Geometry check sheet. Reference: the model listing, model coordinates, mm. Face numbers are marked on the shaded views. A direction names the side the tool comes from. Round coordinates to 2 decimals unless told otherwise and drop trailing zeros. Write each loop counter-clockwise with the first axis right and the second up, starting at its lowest first coordinate (ties: lowest second). Pieces come first, ordered by that corner, then holes. Notation, with made-up numbers: M 83,60.25 L 90,60.25 A13 ccw 90,71.25 Z; hole C 59.25,18.5 d7. An arc over 180 degrees is marked long. Put each result on its own line as item: value. Start each with the question number.
(1) Gauge pin test, flat ends, axial feed: pin 1 (1.1 mm diameter, centred on x = 28.5, z = -20, fed in from +Y); pin 2 (3 mm diameter, centred on x = -14, z = 20, fed in from -Y); pin 3 (0.9 mm diameter, centred on y = 11.5, z = 28, fed in from -X); pin 4 (2 mm diameter, centred on x = 14, z = 23.5, fed in from +Y). Record the tip position at first contact, or that the pin passes through.
(2) Material ranges on probe 1 along X at (y, z) = (7.5, 3); probe 2 along Z at (x, y) = (-43.5, 9.75); probe 3 along Z at (x, y) = (43.5, 16), recorded low to high.
(3) Tool access check on the marked faces 5 and 6. Record the directions out of +Z, -Z, +X, -X, +Y, -Y that give a thin tool (end or side, any length) a straight path to the whole face; none if there is none.
(4) Section check C-C on x = 48.5. Record the cut outline in (y, z), then the cut area to 3 significant figures.
(5) Section check B-B on x = -11.1. Record the cut outline in (y, z), then the cut area to 3 significant figures.
(6) Section check A-A on x = 14. Record the cut outline in (y, z).
(7) Mould release check, pull along Z, two halves, no side actions. Record for the marked faces 1, 2, 3 and 4: pulls with the +Z half, pulls with the -Z half, needs draft (parallel to the pull), parting line crosses it, or undercut.
from build123d import *

# Parameters (mm, degrees)
BOSS_EXTRUDE1_DEPTH = 2
BOSS_EXTRUDE2_DEPTH = 16
SKETCH12_W          = 7
SKETCH12_H          = 7
BOSS_EXTRUDE5_DEPTH = 16
FILLET1_R           = 3
SKETCH13_R          = 1.3
CUT_EXTRUDE7_DEPTH  = 19
SKETCH14_R          = 2.5
SKETCH14_R_2        = 1.15
BOSS_EXTRUDE6_DEPTH = 14
SKETCH15_R          = 2.5
SKETCH15_R_2        = 1.3
BOSS_EXTRUDE7_DEPTH = 3
SKETCH16_W          = 9
SKETCH16_H          = 4.5
CUT_EXTRUDE8_DEPTH  = 4
SKETCH17_R          = 3.25
CUT_EXTRUDE9_DEPTH  = 13
SKETCH19_R          = 2.5
SKETCH19_R_2        = 1.15
BOSS_EXTRUDE8_DEPTH = 2.5
SKETCH20_R          = 3.1
SKETCH20_R_2        = 3
SKETCH20_W          = 4
SKETCH20_H          = 11
CUT_EXTRUDE10_DEPTH = 5
SKETCH21_R          = 1.15
CUT_EXTRUDE11_DEPTH = 3.5
SKETCH22_R          = 1.15
CUT_EXTRUDE12_DEPTH = 3.5


with BuildPart() as part:
    # Sketch1 → Boss-Extrude1 (new body)
    with BuildSketch(Plane(origin=(0, 0, 0), x_dir=(1, 0, 0), z_dir=(0, 1, 0))):
        with BuildLine():
            Line((70, 10), (70, -10))
            ThreePointArc((70, -10), (64.142135624, -24.142135624), (50, -30))
            Line((50, -30), (-50, -30))
            ThreePointArc((-50, -30), (-64.142135624, -24.142135624), (-70, -10))
            Line((-70, -10), (-70, 10))
            ThreePointArc((-70, 10), (-64.142135624, 24.142135624), (-50, 30))
            Line((-50, 30), (50, 30))
            ThreePointArc((50, 30), (64.142135624, 24.142135624), (70, 10))
        make_face()
    extrude(amount=BOSS_EXTRUDE1_DEPTH)

    # Sketch2 → Boss-Extrude2 (add)
    with BuildSketch(Plane(origin=(0, 2, 0), x_dir=(1, 0, 0), z_dir=(0, 1, 0))):
        with BuildLine():
            Line((-50, 30), (50, 30))
            ThreePointArc((50, 30), (64.142135624, 24.142135624), (70, 10))
            Line((70, 10), (70, -10))
            ThreePointArc((70, -10), (64.142135624, -24.142135624), (50, -30))
            Line((50, -30), (-50, -30))
            ThreePointArc((-50, -30), (-64.142135624, -24.142135624), (-70, -10))
            Line((-70, -10), (-70, 10))
            ThreePointArc((-70, 10), (-64.142135624, 24.142135624), (-50, 30))
        make_face()
        with BuildLine():
            Line((-47, 27), (47, 27))
            ThreePointArc((47, 27), (60.435028843, 21.435028843), (66, 8))
            Line((66, 8), (66, -12))
            ThreePointArc((66, -12), (59.103718437, -22.798043353), (47, -27))
            Line((47, -27), (-47, -27))
            ThreePointArc((-47, -27), (-59.103718437, -22.798043353), (-66, -12))
            Line((-66, -12), (-66, 8))
            ThreePointArc((-66, 8), (-60.435028843, 21.435028843), (-47, 27))
        make_face(mode=Mode.SUBTRACT)
    extrude(amount=BOSS_EXTRUDE2_DEPTH)

    # Sketch12 → Boss-Extrude5 (add)
    with BuildSketch(Plane(origin=(0, 2, 0), x_dir=(1, 0, 0), z_dir=(0, 1, 0))):
        with Locations((-43.5, 23.5)):
            Rectangle(SKETCH12_W, SKETCH12_H)
        with Locations((-43.5, -23.5)):
            Rectangle(SKETCH12_W, SKETCH12_H)
        with Locations((43.5, -23.5)):
            Rectangle(SKETCH12_W, SKETCH12_H)
        with Locations((43.5, 23.5)):
            Rectangle(SKETCH12_W, SKETCH12_H)
    extrude(amount=BOSS_EXTRUDE5_DEPTH)

    # Fillet1
    fillet1_edges = [part.edges().sort_by_distance(p)[0] for p in [
        (70, 0, 0),
        (64.142135624, 0, 24.142135624),
        (0, 0, 30),
        (-64.142135624, 0, 24.142135624),
        (-70, 0, 0),
        (-64.142135624, 0, -24.142135624),
        (0, 0, -30),
        (64.142135624, 0, -24.142135624),
    ]]
    fillet(fillet1_edges, radius=FILLET1_R)

    # Sketch13 → Cut-Extrude7 (cut, through all)
    with BuildSketch(Plane(origin=(0, 18, 0), x_dir=(1, 0, 0), z_dir=(0, 1, 0))):
        with Locations((-43.5, 23.5)):
            Circle(SKETCH13_R)
        with Locations((-43.5, -23.5)):
            Circle(SKETCH13_R)
        with Locations((43.5, -23.5)):
            Circle(SKETCH13_R)
        with Locations((43.5, 23.5)):
            Circle(SKETCH13_R)
    extrude(amount=-CUT_EXTRUDE7_DEPTH, mode=Mode.SUBTRACT)

    # Sketch14 → Boss-Extrude6 (add)
    with BuildSketch(Plane(origin=(0, 2, 0), x_dir=(1, 0, 0), z_dir=(0, 1, 0))):
        with Locations((29, -3)):
            Circle(SKETCH14_R)
        with Locations((29, -3)):
            Circle(SKETCH14_R_2, mode=Mode.SUBTRACT)
        with Locations((29, 20)):
            Circle(SKETCH14_R)
        with Locations((29, 20)):
            Circle(SKETCH14_R_2, mode=Mode.SUBTRACT)
        with Locations((-29, 20)):
            Circle(SKETCH14_R)
        with Locations((-29, 20)):
            Circle(SKETCH14_R_2, mode=Mode.SUBTRACT)
        with Locations((-29, -3)):
            Circle(SKETCH14_R)
        with Locations((-29, -3)):
            Circle(SKETCH14_R_2, mode=Mode.SUBTRACT)
    extrude(amount=BOSS_EXTRUDE6_DEPTH)

    # Sketch15 → Boss-Extrude7 (add)
    with BuildSketch(Plane(origin=(0, 2, 0), x_dir=(1, 0, 0), z_dir=(0, 1, 0))):
        with Locations((29, -23)):
            Circle(SKETCH15_R)
        with Locations((29, -23)):
            Circle(SKETCH15_R_2, mode=Mode.SUBTRACT)
        with Locations((14, -23)):
            Circle(SKETCH15_R)
        with Locations((14, -23)):
            Circle(SKETCH15_R_2, mode=Mode.SUBTRACT)
    extrude(amount=BOSS_EXTRUDE7_DEPTH)

    # Sketch16 → Cut-Extrude8 (cut, through all)
    with BuildSketch(Plane(origin=(0, 0, 27), x_dir=(-1, 0, 0), z_dir=(0, 0, -1))):
        with Locations((-20.5, 7.75)):
            Rectangle(SKETCH16_W, SKETCH16_H)
    extrude(amount=-CUT_EXTRUDE8_DEPTH, mode=Mode.SUBTRACT)

    # Sketch17 → Cut-Extrude9 (cut)
    with BuildSketch(Plane.XZ):
        with Locations((-43.5, 23.5)):
            Circle(SKETCH17_R)
        with Locations((43.5, 23.5)):
            Circle(SKETCH17_R)
        with Locations((43.5, -23.5)):
            Circle(SKETCH17_R)
        with Locations((-43.5, -23.5)):
            Circle(SKETCH17_R)
    extrude(amount=-CUT_EXTRUDE9_DEPTH, mode=Mode.SUBTRACT)

    # Sketch19 → Boss-Extrude8 (add)
    with BuildSketch(Plane(origin=(0, 0, 27), x_dir=(-1, 0, 0), z_dir=(0, 0, -1))):
        with Locations((-1, 9)):
            Circle(SKETCH19_R)
        with Locations((-1, 9)):
            Circle(SKETCH19_R_2, mode=Mode.SUBTRACT)
        with Locations((34, 9)):
            Circle(SKETCH19_R)
        with Locations((34, 9)):
            Circle(SKETCH19_R_2, mode=Mode.SUBTRACT)
    extrude(amount=BOSS_EXTRUDE8_DEPTH)

    # Sketch20 → Cut-Extrude10 (cut)
    with BuildSketch(Plane(origin=(0, 0, 27), x_dir=(-1, 0, 0), z_dir=(0, 0, -1))):
        with Locations((11.1, 9)):
            Circle(SKETCH20_R)
        with Locations((25, 9)):
            Circle(SKETCH20_R_2)
        with Locations((5, 9)):
            Rectangle(SKETCH20_W, SKETCH20_H)
    extrude(amount=-CUT_EXTRUDE10_DEPTH, mode=Mode.SUBTRACT)

    # Sketch21 → Cut-Extrude11 (cut)
    with BuildSketch(Plane(origin=(0, 0, 24.5), x_dir=(-1, 0, 0), z_dir=(0, 0, -1))):
        with Locations((-1, 9)):
            Circle(SKETCH21_R)
    extrude(amount=-CUT_EXTRUDE11_DEPTH, mode=Mode.SUBTRACT)

    # Sketch22 → Cut-Extrude12 (cut)
    with BuildSketch(Plane(origin=(0, 0, 24.5), x_dir=(-1, 0, 0), z_dir=(0, 0, -1))):
        with Locations((34, 9)):
            Circle(SKETCH22_R)
    extrude(amount=-CUT_EXTRUDE12_DEPTH, mode=Mode.SUBTRACT)


solid = part.part
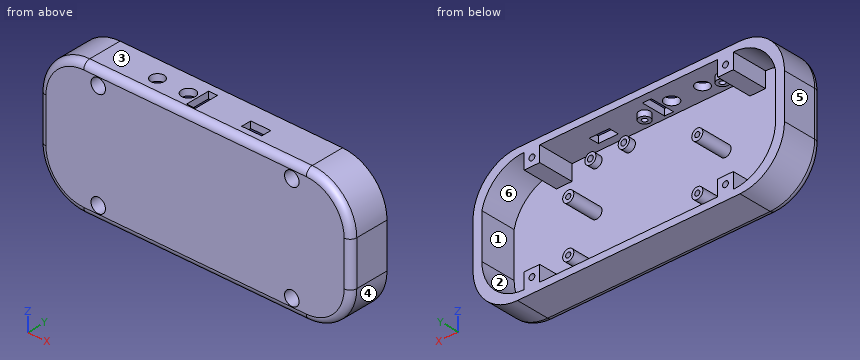
Answers follow:
1. pin 1: stops at y = 2
1. pin 2: stops at y = 0
1. pin 3: stops at x = -59.59
1. pin 4: stops at y = 5
2. probe 1: x = -70 to -66, -31.5 to -30.15, -27.85 to -26.5, 26.5 to 27.85, 30.15 to 31.5, 66 to 70
2. probe 2: z = -30 to -26.75, -20.25 to -20, 20 to 20.25, 26.75 to 30
2. probe 3: z = -30 to -24.8, -22.2 to -20, 20 to 22.2, 24.8 to 30
3. face 5: +Z, -Z, -X, +Y, -Y
3. face 6: +Y
4. outline: M 0,-27 A3 ccw 3,-30 L 18,-30 L 18,-26.94 L 2,-26.94 L 2,26.94 L 18,26.94 L 18,30 L 3,30 A3 ccw 0,27 Z
4. area: 214 mm^2
5. outline: M 0,-27 A3 ccw 3,-30 L 18,-30 L 18,-27 L 2,-27 L 2,27 L 5.9,27 L 5.9,30 L 3,30 A3 ccw 0,27 Z; M 12.1,27 L 18,27 L 18,30 L 12.1,30 Z
5. area: 194 mm^2
6. outline: M 0,-27 A3 ccw 3,-30 L 18,-30 L 18,-27 L 2,-27 L 2,20.5 L 5,20.5 L 5,21.7 L 2,21.7 L 2,24.3 L 5,24.3 L 5,25.5 L 2,25.5 L 2,27 L 18,27 L 18,30 L 3,30 A3 ccw 0,27 Z
7. face 1: undercut
7. face 2: undercut
7. face 3: pulls with the +Z half
7. face 4: pulls with the -Z half
